from build123d import *

# Parameters (mm, degrees)
SKIZZE1_R                            = 9.6
AUFSATZ_LINEAR_AUSTRAGEN1_DEPTH      = 10.3
AUFSATZ_LINEAR_AUSTRAGEN1_DEPTH_BACK = 10.3
SKIZZE2_R                            = 11.1
AUFSATZ_LINEAR_AUSTRAGEN2_DEPTH      = 1.8
SKIZZE3_R                            = 11.1
AUFSATZ_LINEAR_AUSTRAGEN3_DEPTH      = 1.8
FASE1_SIZE                           = 0.5


with BuildPart() as part:
    # Skizze1 → Aufsatz-Linear austragen1 (new body, two sides)
    with BuildSketch(Plane.XY) as aufsatz_linear_austragen1_sk:
        Circle(SKIZZE1_R)
    extrude(amount=AUFSATZ_LINEAR_AUSTRAGEN1_DEPTH)
    extrude(aufsatz_linear_austragen1_sk.sketch, amount=-AUFSATZ_LINEAR_AUSTRAGEN1_DEPTH_BACK)

    # Skizze2 → Aufsatz-Linear austragen2 (add)
    with BuildSketch(Plane.XY.offset(10.3)):
        Circle(SKIZZE2_R)
    extrude(amount=-AUFSATZ_LINEAR_AUSTRAGEN2_DEPTH)

    # Skizze3 → Aufsatz-Linear austragen3 (add)
    with BuildSketch(Plane(origin=(0, 0, -10.3), x_dir=(-1, 0, 0), z_dir=(0, 0, -1))):
        Circle(SKIZZE3_R)
    extrude(amount=-AUFSATZ_LINEAR_AUSTRAGEN3_DEPTH)

    # Skizze8 → Schnitt-Rotation1 (revolve, cut)
    with BuildSketch(Plane(origin=(0, 0, 0), x_dir=(0, 0, -1), z_dir=(1, 0, 0))):
        Polygon((10.3, 0), (10.3, 8), (8.5, 8), (-2.7, 6), (-2.7, 1.5), (-6.3, 1.5), (-6.3, 4.1), (-10.3, 4.1), (-10.3, 0), align=None)
    revolve(axis=Axis((0, 0, -9.8), (0, 0, 1)), mode=Mode.SUBTRACT)

    # Fase1
    fase1_edges = [part.edges().sort_by_distance(p)[0] for p in [
        (0, -1.5, 2.7),
        (0, -1.5, 6.3),
        (0, -4.1, 10.3),
    ]]
    chamfer(fase1_edges, length=FASE1_SIZE)


solid = part.part
The model under review builds one solid part; all positions refer to its coordinate system, in mm. A direction names the side the tool comes from. Coordinates: 2 decimals unless noted, no trailing zeros. Write each loop counter-clockwise with the first axis right and the second up, starting at its lowest first coordinate (ties: lowest second). Pieces come first, ordered by that corner, then holes. Notation, with made-up numbers: (51, 18) -> (102, 18) arc R14 ccw to (102, 33) -> close; hole circle Ø1 at (4, -40). An arc over 180 degrees is marked (long way). Answer in a Markdown table with one row per item.
1. Wall thickness on probe 1 along Z at (x, y) = (8.5, -5); probe 2 along Y at (x, z) = (0, 7.5); probe 3 along Y at (x, z) = (0, -9.3): over which ranges is each line inside the solid? List them lowest first. Write a range as [from, to].
Answers below:
| item | result |
|---|---|
| probe 1 | z = [-10.3, -8.5], [8.5, 10.3] |
| probe 2 | y = [-9.6, -4.1], [4.1, 9.6] |
| probe 3 | y = [-11.1, -8], [8, 11.1] |
2. We need section D-D, the plane y = 8.75. State the section outline as (x, z) points.
Answers below:
| item | result |
|---|---|
| outline | (-6.83, -10.3) -> (6.83, -10.3) -> (6.83, -8.5) -> (3.95, -8.5) -> (3.95, 8.5) -> (6.83, 8.5) -> (6.83, 10.3) -> (-6.83, 10.3) -> (-6.83, 8.5) -> (-3.95, 8.5) -> (-3.95, -8.5) -> (-6.83, -8.5) -> close |
3. We need section C-C, the plane z = -2.5. State the section outline as (x, y) points, and give its area (3 significant figures).
Answers below:
| item | result |
|---|---|
| outline | circle Ø19.2 at (0, 0); hole circle Ø13.86 at (0, 0) |
| area | 139 mm^2 |
4. Clearance check with flat-ended pins moving along their axes: pin 1 Ø12 at (y, z) = (-4.5, -2) entering from +X; pin 2 Ø2 at (y, z) = (-4, -8) entering from -X; pin 3 Ø1.5 at (y, z) = (5, -5) entering from +X; pin 4 Ø6.5 at (x, y) = (-1.5, 0.5) entering from +Z. State where each tip first meets the part, or that it passes through.
Answers below:
| item | result |
|---|---|
| pin 1 | stops at x = 9.6 |
| pin 2 | stops at x = -10.65 |
| pin 3 | stops at x = 8.61 |
| pin 4 | stops at z = 10.3 |
5. Draft analysis for pull direction Z (two halves, no side actions). For faces 6 (the flat face through (7, 7, -8.5)), 7 (the flat face through (5, 0, 10.3)), 8 (the cylindrical face through (-5.97, 9.36, -9.41)), state which applies: +Z half, -Z half, draft (parallel to the pull), parting line (faces both ways), or undercut.
Answers below:
| item | result |
|---|---|
| face 6 | undercut |
| face 7 | +Z half |
| face 8 | draft |
6. For faces 1 (the flat face through (-6, 6, -10.3)), 2 (the cylindrical face through (7.81, -1.73, -9.39)), 3 (the cylindrical face through (5.97, 9.36, 9.41)), 4 (the flat face through (2, 1, 6.3)), 5 (the cylindrical face through (5.161, 8.095, 0.119)), list the 3-axis set-ups (+Z, -Z, +X, -X, +Y, -Y) from which the entire face can be reached by the end or side of a thin tool; tool diameter is ignored.
Answers below:
| item | result |
|---|---|
| face 1 | -Z, +X, -X, +Y, -Y |
| face 2 | -Z |
| face 3 | +Z, -Z |
| face 4 | +Z |
| face 5 | none |
